The model under review builds one solid part; all positions refer to its coordinate system, in mm. Face numbers are marked on the shaded views. A direction names the side the tool comes from. Coordinates: 2 decimals unless noted, no trailing zeros. Write each loop counter-clockwise with the first axis right and the second up, starting at its lowest first coordinate (ties: lowest second). Pieces come first, ordered by that corner, then holes.
1) For P1, Ø4, axis at x = 10.5, z = 184.5, coming from the +Y side; P2, Ø3, axis at y = 360, z = 115.5, coming from the +X side; P3, Ø4, axis at x = 7, y = 86, coming from the -Z side; P4, Ø1, axis at x = -9, z = 254.5, coming from the -Y side, all flat-tipped, find the tip position at first contact; note any pin that passes through.
2) For line 1 (X direction, y = 26, z = 0); line 2 (Y direction, x = 0, z = 431); line 3 (Z direction, x = 0, y = 57), list the stretches that pass through material, from the lowest coordinate up.
3) Machinability: for the marked faces 1 and 2, which of the approach directions +Z, -Z, +X, -X, +Y, -Y give a long, thin tool a straight path to every point of the face, cutting with its end or side? Answer none if there is none.
4) Add section A-A, the plane x = 0. State the section outline as (y, z) points, then the cut area to 3 significant figures.
from build123d import *

# Parameters (mm, degrees)
F0_R   = 19
F0_R_2 = 15.5


with BuildPart() as f2:
    # F2: sweep along a path in F1
    with BuildLine(Plane.YZ) as f2_path:
        Line((0, 0), (50, 0))
        ThreePointArc((50, 0), (332.8427124746, 117.1572875254), (450, 400))
        Line((450, 400), (450, 450))
    # F0 (on Front) → F2 (sweep)
    with BuildSketch(Plane.XZ):
        Circle(F0_R)
        Circle(F0_R_2, mode=Mode.SUBTRACT)
    sweep(path=f2_path.line)


solid = f2.part
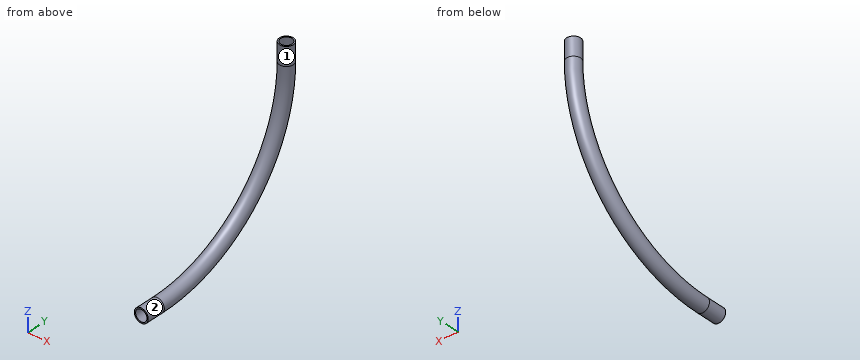
Geometry results:
1. P1: stops at y = 407.49
1. P2: passes through
1. P3: stops at z = -16.8
1. P4: stops at y = 404.23
2. line 1: x = -19 to -15.5, 15.5 to 19
2. line 2: y = 431 to 434.5, 465.5 to 469
2. line 3: z = -18.94 to -15.44, 15.56 to 19.06
3. face 1: +Z
3. face 2: -Y
4. outline: (0, -19) - (50, -19) arc R419 ccw to (469, 400) - (469, 450) - (465.5, 450) - (465.5, 400) arc R415.5 cw to (50, -15.5) - (0, -15.5) - close; (0, 15.5) - (50, 15.5) arc R384.5 ccw to (434.5, 400) - (434.5, 450) - (431, 450) - (431, 400) arc R381 cw to (50, 19) - (0, 19) - close
4. area: 5,100 mm2
